from build123d import *

# Parameters (mm, degrees)
BOSS_EXTRUDE2_DEPTH = 5
SKETCH3_R           = 3.25
CUT_EXTRUDE1_DEPTH  = 11
SKETCH4_W           = 13
SKETCH4_H           = 7
BOSS_EXTRUDE3_DEPTH = 2.5
SKETCH5_R           = 2.5
CUT_EXTRUDE2_DEPTH  = 8.5


with BuildPart() as part:
    # Sketch2 → Boss-Extrude2 (new body, symmetric)
    with BuildSketch(Plane.XY):
        Polygon((0, 0), (-7, 0), (-17, 10), (-10, 10), align=None)
    extrude(amount=BOSS_EXTRUDE2_DEPTH, both=True)

    # Sketch3 → Cut-Extrude1 (cut, through all)
    with BuildSketch(Plane.XZ):
        with Locations((-3.5, 0)):
            Circle(SKETCH3_R)
    extrude(amount=-CUT_EXTRUDE1_DEPTH, mode=Mode.SUBTRACT)

    # Sketch4 → Boss-Extrude3 (add, symmetric)
    with BuildSketch(Plane.XY):
        with Locations((-16.5, 6.5)):
            Rectangle(SKETCH4_W, SKETCH4_H)
    extrude(amount=BOSS_EXTRUDE3_DEPTH, both=True)

    # Sketch5 → Cut-Extrude2 (cut, through all)
    with BuildSketch(Plane.XY.offset(2.5)):
        with Locations((-20, 6.5)):
            Circle(SKETCH5_R)
    extrude(amount=-CUT_EXTRUDE2_DEPTH, mode=Mode.SUBTRACT)


solid = part.part
Source: CAD feature listing. Evaluate the final solid. Frame: model axes, mm. A direction names the side the tool comes from. Round coordinates to 2 decimals unless told otherwise and drop trailing zeros. Loops run counter-clockwise (first coordinate to the right, second up) from the corner with the lowest first, then second, coordinate; pieces in that order, holes last. Notation, with made-up numbers: M 26,-10.75 L 58,-10.75 A13 cw 58,6.25 Z; hole C -9.75,3 d9. An arc over 180 degrees is marked long. Return JSON: item names as keys, results as strings. Group by question number.
1. Section query A-A on z = 0. Output: boundary loops of the cut face in (x, y), and give its area (3 significant figures).
2. Section query C-C on y = 6.5. Output: boundary loops of the cut face in (x, z).
3. Material intervals for line 1 along Z through (x, y) = (-3.5, 1.75); line 2 along Y through (x, z) = (-20, 0.3); line 3 along Y through (x, z) = (-19.5, -1.5), sorted ascending. Write a range as from..to.
4. Mould query, pull axis Y, two halves, no side actions, for faces 1 (the face through (-7, 7, 0)), 2 (the face through (-22.5, 6.6, 0)), 3 (the face through (-17, 6, -2.5)). Classes: released by +Y, released by -Y, zero draft, split by the parting line, or undercut.
5. Section query D-D on z = -3. Output: boundary loops of the cut face in (x, y), and give its area (4 significant figures).
6. Section query B-B on x = -3.5. Output: boundary loops of the cut face in (y, z).
7. Pin query (flat end, axial travel): pin 1 (3 mm diameter, centred on x = -11, y = 1, fed in from -Z); pin 2 (2.5 mm diameter, centred on x = -19, z = 1, fed in from -Y); pin 3 (3.5 mm diameter, centred on x = -17.5, y = 7.5, fed in from +Z); pin 4 (3.5 mm diameter, centred on x = -17, y = 6.5, fed in from -Z). Return the tip coordinate at first contact, or that it passes through.
8. Reachability of faces 4 (the face through (-17, 3, 0)), 5 (the face through (-15, 10, 0)), 6 (the face through (-17, 6, 2.5)) from +Z, -Z, +X, -X, +Y, -Y: full face, straight path, thin tool, end or side. Return the list, or none.
Checks:
{
 "1": {"outline": "M -23,3 L -10,3 L -7,0 L -6.75,0 L -6.75,6.75 L -10,10 L -23,10 Z; M -0.25,0 L 0,0 L -0.25,0.25 Z; hole C -20,6.5 d5", "area": "94.1 mm²"},
 "2": {"outline": "M -23,-2.5 L -22.5,-2.5 L -22.5,2.5 L -23,2.5 Z; M -17.5,-2.5 L -13.5,-2.5 L -13.5,-5 L -6.5,-5 L -6.5,-1.25 A3.25 cw -6.5,1.25 L -6.5,5 L -13.5,5 L -13.5,2.5 L -17.5,2.5 Z"},
 "3": {"line 1": "z = -5..-3.25, 3.25..5", "line 2": "y = 3..4, 9..10", "line 3": "y = 3..4.05, 8.95..10"},
 "4": {"face 1": "released by +Y", "face 2": "undercut", "face 3": "zero draft"},
 "5": {"outline": "M -17,10 L -7,0 L -4.75,0 L -4.75,4.75 L -10,10 Z; M -2.25,0 L 0,0 L -2.25,2.25 Z", "area": "61.25 mm²"},
 "6": {"outline": "M 0,-5 L 3.5,-5 L 3.5,-3.25 L 0,-3.25 Z; M 0,3.25 L 3.5,3.25 L 3.5,5 L 0,5 Z"},
 "7": {"pin 1": "passes through", "pin 2": "stops at y = 3", "pin 3": "stops at z = 2.5", "pin 4": "stops at z = -2.5"},
 "8": {"face 4": "+Z, -Z, -X, -Y", "face 5": "+Z, -Z, +X, -X, +Y", "face 6": "+Z, -X, -Y"}
}
